Geometry: final body of the model. Coordinates: model frame, mm. A direction names the side the tool comes from. Coordinates: 2 decimals unless noted, no trailing zeros. Write each loop counter-clockwise with the first axis right and the second up, starting at its lowest first coordinate (ties: lowest second). Pieces come first, ordered by that corner, then holes. Notation, with made-up numbers: M -21,2.5 L 25,2.5 A18 ccw 25,10.5 Z; hole C 60.5,15.5 d4. An arc over 180 degrees is marked long. Write item = value, one per line. Start each with the question number.
Item 1: Pull-direction query (Y, two-part tool) for faces 3 (the flat face through (27, -5.401, 2)), 4 (the flat face through (27, -5, 3)), 5 (the flat face through (28, -30, 1)), 6 (the flat face through (57.362, -15, 2)); classes: +Y half, -Y half, draft (parallel to the pull), parting line (faces both ways), or undercut.
Item 2: Section A-A on x = 56. Output: boundary loops of the cut face in (y, z).
Item 3: Section B-B on y = -16.5. Output: boundary loops of the cut face in (x, z), plus the area to 3 significant figures.
Item 4: Ray query, L1, parallel to Y at x = 56.5, z = 0.7; L2, parallel to X at y = -11.75, z = 1.75. Return the intervals inside material, ascending. Write a range as [from, to].
Item 5: Reachability of faces 1 (the flat face through (-2.638, -16, 2)), 2 (the flat face through (27, -5, 0)) from +Z, -Z, +X, -X, +Y, -Y: full face, straight path, thin tool, end or side. Return the list, or none.
Item 6: Section C-C on z = 0.65. Output: boundary loops of the cut face in (x, y).
Autodesk Inventor part; units mm, degrees
ref_plane "YZ Plane" through (0, 0, 0) normal (1, 0, 0) x (0, 1, 0)
ref_plane "XZ Plane" through (0, 0, 0) normal (0, 1, 0) x (-1, 0, 0)
ref_plane "XY Plane" through (0, 0, 0) normal (0, 0, 1) x (1, 0, 0)
sketch "Sketch1" plane through (0, 0, 0) normal (0, 0, 1) x (1, 0, 0)
  line L0 (-7.1091, 0) -> (62.8909, 0)
  line L1 (62.8909, 0) -> (62.8909, -30)
  line L2 (62.8909, -30) -> (-7.1091, -30)
  line L3 (-7.1091, -30) -> (-7.1091, 0)
  point P0 (0, 0)
  dimension "d0" = 70
  dimension "d1" = 30
extrude "Extrusion1" add sketch "Sketch1" along normal blind 3
sketch "Sketch2" plane through (0, 0, 3) normal (0, 0, 1) x (1, 0, 0)
  line L0 (57.3616, -25.4008) -> (-2.6384, -25.4008)
  line L1 (-2.6384, -25.4008) -> (-2.6384, -5.4008)
  line L2 (-2.6384, -5.4008) -> (57.3616, -5.4008)
  line L3 (57.3616, -5.4008) -> (57.3616, -25.4008)
  line L4 (57.3616, -25.4008) -> (-2.6384, -5.4008) construction
  line L5 (-2.6384, -25.4008) -> (57.3616, -5.4008) construction
  point P0 (0, 0)
  point P1 (27.3616, -15.4008)
  dimension "d4" = 60
  dimension "d5" = 20
extrude "Extrusion2" cut sketch "Sketch2" against normal blind 3
properties part number "mouth_open"
Responses:
q1.face_3 = undercut
q1.face_4 = draft
q1.face_5 = -Y half
q1.face_6 = undercut
q2.outline = M -30,0 L -25.4,0 L -25.4,3 L -30,3 Z; M -5.4,0 L 0,0 L 0,3 L -5.4,3 Z
q3.outline = M -7.11,0 L -2.64,0 L -2.64,3 L -7.11,3 Z; M 57.36,0 L 62.89,0 L 62.89,3 L 57.36,3 Z
q3.area = 30.0 mm²
q4.L1 = [-30, -25.4], [-5.4, 0]
q4.L2 = [-7.11, -2.64], [57.36, 62.89]
q5.face_1 = +Z, -Z
q5.face_2 = -Z, +X, -X, +Y, -Y
q6.outline = M -7.11,-30 L 62.89,-30 L 62.89,0 L -7.11,0 Z; hole M -2.64,-25.4 L 57.36,-25.4 L 57.36,-5.4 L -2.64,-5.4 Z
